Verification items for the finished model (mm, model axes). A direction names the side the tool comes from. Coordinates: 2 decimals unless noted, no trailing zeros. Order: outer loops, then holes, each group sorted by start corner. A loop starts at its lowest first (then second) coordinate and runs counter-clockwise, first axis right, second up. Notation, with made-up numbers: M -18,-36.75 L 41,-36.75 A26 ccw 41,-12.75 Z; hole C -32.5,86.25 d10. An arc over 180 degrees is marked long. Write item = value, one per line.
```python
from build123d import *

# Parameters (mm, degrees)
SKETCH1_W               = 40
SKETCH1_H               = 36
BOSS_EXTRUDE1_DEPTH     = 10
BOSS_EXTRUDE2_START     = 7.62
SKETCH2_W               = 7
SKETCH2_H               = 20
BOSS_EXTRUDE2_DEPTH     = 2
CUT_EXTRUDE1_DEPTH      = 34.955853693
CUT_EXTRUDE1_DEPTH_BACK = 34.955853693
FILLET1_R               = 0.254
BOSS_EXTRUDE4_START     = 18
SKETCH5_R               = 2.921
BOSS_EXTRUDE4_DEPTH     = 8.704


with BuildPart() as part:
    # Sketch1 → Boss-Extrude1 (new, symmetric)
    with BuildSketch(Plane(origin=(0, 0, 0), x_dir=(1, 0, 0), z_dir=(0, 1, 0))):
        Rectangle(SKETCH1_W, SKETCH1_H)
    extrude(amount=BOSS_EXTRUDE1_DEPTH, both=True)

    # Sketch2 → Boss-Extrude2 (add)
    with BuildSketch(Plane.XY.offset(BOSS_EXTRUDE2_START)):
        with Locations((-23.5, 0)):
            Rectangle(SKETCH2_W, SKETCH2_H)
        with Locations((23.5, 0)):
            Rectangle(SKETCH2_W, SKETCH2_H)
    extrude(amount=BOSS_EXTRUDE2_DEPTH)

    # Sketch4 → Cut-Extrude1 (cut, two sides: drawn at the far end of the back side and taken through both)
    with BuildSketch(Plane.XY.offset(-CUT_EXTRUDE1_DEPTH_BACK)):
        with BuildLine():
            Line((-27, 5.393), (-26.739840954, 5.393))
            ThreePointArc((-26.739840954, 5.393), (-22.225, 4.885), (-26.739840954, 4.377))
            Line((-26.739840954, 4.377), (-27, 4.377))
            Line((-27, 4.377), (-27, 5.393))
        make_face()
        with BuildLine():
            Line((27, 4.377), (26.739840954, 4.377))
            ThreePointArc((26.739840954, 4.377), (22.225, 4.885), (26.739840954, 5.393))
            Line((26.739840954, 5.393), (27, 5.393))
            Line((27, 5.393), (27, 4.377))
        make_face()
        with BuildLine():
            Line((27, -5.393), (26.739840954, -5.393))
            ThreePointArc((26.739840954, -5.393), (22.225, -4.885), (26.739840954, -4.377))
            Line((26.739840954, -4.377), (27, -4.377))
            Line((27, -4.377), (27, -5.393))
        make_face()
        with BuildLine():
            Line((-27, -4.377), (-26.739840954, -4.377))
            ThreePointArc((-26.739840954, -4.377), (-22.225, -4.885), (-26.739840954, -5.393))
            Line((-26.739840954, -5.393), (-27, -5.393))
            Line((-27, -5.393), (-27, -4.377))
        make_face()
    extrude(amount=CUT_EXTRUDE1_DEPTH + CUT_EXTRUDE1_DEPTH_BACK, mode=Mode.SUBTRACT)

    # Fillet1
    # the kernel refuses this fillet: 0.254 mm, written as the material it takes off along each edge
    with BuildSketch(Plane(origin=(26.739840954, -5.393, 7.134588457), x_dir=(1, 0, 0), z_dir=(0, 0, 1)), Plane(origin=(26.739840954, 4.377, 7.134588457), x_dir=(1, 0, 0), z_dir=(0, 0, 1))) as fillet1_piece_1:
        with BuildLine():
            CenterArc((0.194164617, -0.254), FILLET1_R, 90, 72.542396876)
            ThreePointArc((-0.04813594, -0.1778), (-0.022276402, -0.089385033), (0, 0))
            Line((0, 0), (0.194164617, 0))
        make_face()
    extrude(amount=2.970823086, mode=Mode.SUBTRACT)
    with BuildSketch(Plane(origin=(27, -4.377, 10.255), x_dir=(-1, 0, 0), z_dir=(0, 0, -1)), Plane(origin=(-27, 5.393, 10.255), x_dir=(0, 1, 0), z_dir=(0, 0, -1)), Plane(origin=(27, 4.377, 10.255), x_dir=(0, -1, 0), z_dir=(0, 0, -1)), Plane(origin=(27, -5.393, 10.255), x_dir=(0, -1, 0), z_dir=(0, 0, -1))) as fillet1_piece_2:
        with BuildLine():
            CenterArc((FILLET1_R, FILLET1_R), FILLET1_R, 180, 90)
            Line((0, FILLET1_R), (0, 0))
            Line((0, 0), (FILLET1_R, 0))
        make_face()
    extrude(amount=3.27, mode=Mode.SUBTRACT)
    with BuildSketch(Plane(origin=(26.739840954, 5.393, 7.134588457), x_dir=(-0.2613232863533324, 0.9652513351503299, 0), z_dir=(0, 0, 1)), Plane(origin=(26.739840954, -4.377, 7.134588457), x_dir=(-0.26132328635333724, 0.9652513351503285, 0), z_dir=(0, 0, 1))) as fillet1_piece_3:
        with BuildLine():
            CenterArc((0.194434103, -0.253793771), FILLET1_R, 92.309007358, 72.542396876)
            Line((-0.050739736, -0.187417656), (0, 0))
            ThreePointArc((0, 0), (0.092100365, -0.001856063), (0.184200729, 0))
        make_face()
    extrude(amount=2.970823086, mode=Mode.SUBTRACT)
    with BuildSketch(Plane(origin=(-27, -5.393, 10.255), x_dir=(0, -1, 0), z_dir=(0, 0, -1)), Plane(origin=(-27, -4.377, 10.255), x_dir=(1, 0, 0), z_dir=(0, 0, -1)), Plane(origin=(-27, 4.377, 10.255), x_dir=(0, -1, 0), z_dir=(0, 0, -1)), Plane(origin=(27, 5.393, 10.255), x_dir=(0, 1, 0), z_dir=(0, 0, -1))) as fillet1_piece_4:
        with BuildLine():
            CenterArc((FILLET1_R, -FILLET1_R), FILLET1_R, 90, 90)
            Line((0, -FILLET1_R), (0, 0))
            Line((0, 0), (FILLET1_R, 0))
        make_face()
    extrude(amount=3.27, mode=Mode.SUBTRACT)
    with BuildSketch(Plane(origin=(-26.739840954, -5.393, 7.134588457), x_dir=(-1, 0, 0), z_dir=(0, 0, 1)), Plane(origin=(-26.739840954, 4.377, 7.134588457), x_dir=(-1, 0, 0), z_dir=(0, 0, 1))) as fillet1_piece_5:
        with BuildLine():
            CenterArc((0.194164617, 0.254), FILLET1_R, 197.457603124, 72.542396876)
            ThreePointArc((-0.04813594, 0.1778), (-0.022276402, 0.089385033), (0, 0))
            Line((0, 0), (0.194164617, 0))
        make_face()
    extrude(amount=2.970823086, mode=Mode.SUBTRACT)
    with BuildSketch(Plane(origin=(-26.739840954, -4.377, 7.134588457), x_dir=(0.2613232863533336, 0.9652513351503295, 0), z_dir=(0, 0, 1)), Plane(origin=(-26.739840954, 5.393, 7.134588457), x_dir=(0.2613232863533336, 0.9652513351503295, 0), z_dir=(0, 0, 1))) as fillet1_piece_6:
        with BuildLine():
            CenterArc((0.194434103, 0.253793771), FILLET1_R, 195.148595765, 72.542396876)
            Line((-0.050739736, 0.187417656), (0, 0))
            ThreePointArc((0, 0), (0.092100365, 0.001856063), (0.184200729, 0))
        make_face()
    extrude(amount=2.970823086, mode=Mode.SUBTRACT)

    # Sketch5 → Boss-Extrude4 (add)
    with BuildSketch(Plane.XY.offset(BOSS_EXTRUDE4_START)):
        with Locations(Location((-9.078, 0, 0), (0, 0, 180))):
            Circle(SKETCH5_R)
    extrude(amount=BOSS_EXTRUDE4_DEPTH)


solid = part.part
```
Item 1: Tool access check on faces 4 (the flat face through (23, 0, 9.62)), 5 (the flat face through (-20, 0, -5)), 6 (the flat face through (-27, 0, 9)), 7 (the flat face through (23, 0, 7.62)), 8 (the flat face through (-24, 0, 9.62)). Record the directions out of +Z, -Z, +X, -X, +Y, -Y that give a thin tool (end or side, any length) a straight path to the whole face; none if there is none.
Report:
face_4 = +Z, +X, +Y, -Y
face_5 = -Z, -X, +Y, -Y
face_6 = +Z, -Z, -X, +Y, -Y
face_7 = -Z, +X, +Y, -Y
face_8 = +Z, -X, +Y, -Y
Item 2: Release check for a two-part mould opening along X. For faces 1 (the flat face through (27, 0, 9)), 2 (the flat face through (-27, 8, 9)), 3 (the cylindrical face through (22.227, -4.976, 8.606)) record: pulls with the +X half, pulls with the -X half, needs draft (parallel to the pull), parting line crosses it, or undercut.
Report:
face_1 = pulls with the +X half
face_2 = pulls with the -X half
face_3 = undercut
Item 3: Sectioned sample at C-C, the plane x = 3.5. Enter the section's corners in (y, z).
Report:
outline = M -10,-18 L 10,-18 L 10,18 L -10,18 Z
Item 4: Sectioned sample at B-B, the plane z = -3. Enter the section's corners in (x, y).
Report:
outline = M -20,-10 L 20,-10 L 20,10 L -20,10 Z
Item 5: Sectioned sample at D-D, the plane z = 21. Enter the section's corners in (x, y).
Report:
outline = C -9.08,0 d5.84
Item 6: Sectioned sample at A-A, the plane y = 0. Enter the section's corners in (x, z).
Report:
outline = M -27,7.62 L -20,7.62 L -20,-18 L 20,-18 L 20,7.62 L 27,7.62 L 27,9.62 L 20,9.62 L 20,18 L -6.16,18 L -6.16,26.7 L -12,26.7 L -12,18 L -20,18 L -20,9.62 L -27,9.62 Z
Item 7: Scan lines: L1, parallel to Z at x = -14.5, y = 5; L2, parallel to X at y = -8.5, z = 5; L3, parallel to Z at x = 21.5, y = 5.5. Record each from-to range of solid material in increasing order. Write a range as from..to.
Report:
L1 = -18..18
L2 = -20..20
L3 = 7.62..9.62
Item 8: Gauge pin test, flat ends, axial feed: pin 1 (2 mm diameter, centred on x = 23.5, y = 0, fed in from +Z); pin 2 (6 mm diameter, centred on x = 9.5, y = 1, fed in from +Z); pin 3 (6 mm diameter, centred on y = 4.5, z = -1, fed in from -X). Record the tip position at first contact, or that the pin passes through.
Report:
pin_1 = 9.62
pin_2 = 18
pin_3 = -20
